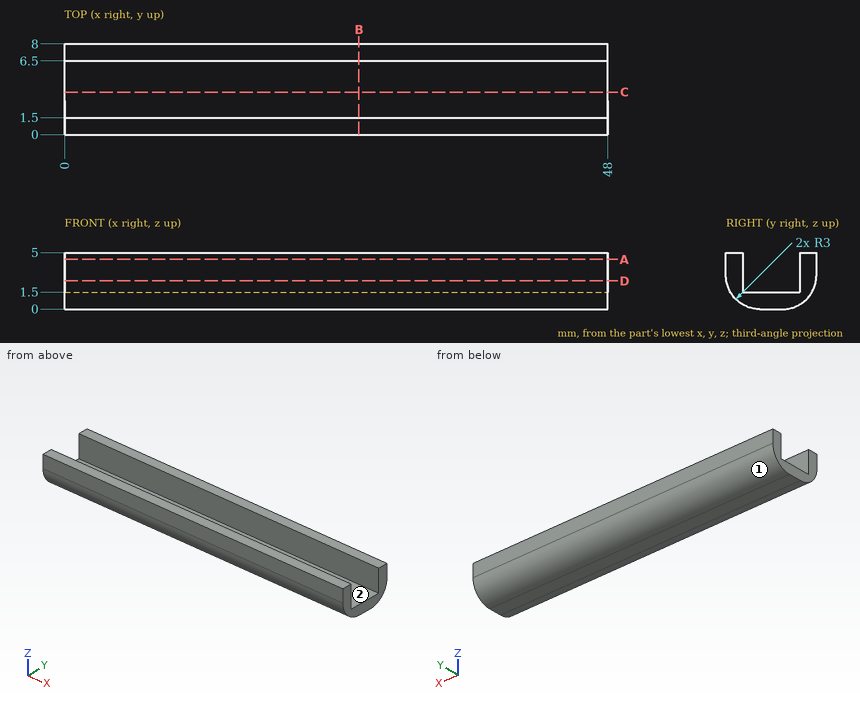
Design review of the part shown in the three views and the two pictorial views. Dimensions are in mm from the part's minimum x, y and z. Round coordinates to 2 decimals unless told otherwise and drop trailing zeros. Write each loop counter-clockwise with the first axis right and the second up, starting at its lowest first coordinate (ties: lowest second). Pieces come first, ordered by that corner, then holes. Notation, with made-up numbers: (64, 85.25) - (117, 85.25) arc R13 cw to (117, 91.25) - close; hole circle Ø6 at (33.25, -18). An arc over 180 degrees is marked (long way). Write item = value, one per line. Start each with the question number.
1. Consider section A-A on z = 4.4. State the section outline as (x, y) points, plus the area to 3 significant figures.
2. For pin 1 Ø2 at (x, y) = (37, 4) entering from +Z; pin 2 Ø3 at (x, z) = (30.5, 2.5) entering from -Y, all flat-tipped, find the tip position at first contact; note any pin that passes through.
3. Consider section D-D on z = 2.5. State the section outline as (x, y) points.
4. Consider section B-B on x = 26. State the section outline as (y, z) points.
5. Draft analysis for pull direction Y (two halves, no side actions). For the marked faces 1 and 2, state which applies: released by +Y, released by -Y, zero draft, split by the parting line, or undercut.
6. Wall thickness on L1, parallel to Y at x = 13.5, z = 4.1; L2, parallel to Z at x = 31, y = 4.25; L3, parallel to Y at x = 45, z = 2.25: over which ranges is each line inside the solid? List them lowest first.
7. Consider section C-C on y = 3.75. State the section outline as (x, z) points.
Evaluation:
q1.outline = (0, 0) - (48, 0) - (48, 1.5) - (0, 1.5) - close; (0, 6.5) - (48, 6.5) - (48, 8) - (0, 8) - close
q1.area = 144 mm2
q2.pin_1 = 1.5
q2.pin_2 = 0
q3.outline = (0, 0.04) - (48, 0.04) - (48, 1.5) - (0, 1.5) - close; (0, 6.5) - (48, 6.5) - (48, 7.96) - (0, 7.96) - close
q4.outline = (0, 3) arc R3 ccw to (3, 0) - (5, 0) arc R3 ccw to (8, 3) - (8, 5) - (6.5, 5) - (6.5, 1.5) - (1.5, 1.5) - (1.5, 5) - (0, 5) - close
q5.face_1 = released by +Y
q5.face_2 = undercut
q6.L1 = 0 to 1.5, 6.5 to 8
q6.L2 = 0 to 1.5
q6.L3 = 0.1 to 1.5, 6.5 to 7.9
q7.outline = (0, 0) - (48, 0) - (48, 1.5) - (0, 1.5) - close
